Input: part model. Units: mm. Frame: model coordinates. A direction names the side the tool comes from. Round coordinates to 2 decimals unless told otherwise and drop trailing zeros. Loops run counter-clockwise (first coordinate to the right, second up) from the corner with the lowest first, then second, coordinate; pieces in that order, holes last. Notation, with made-up numbers: (55, 8) - (90, 8) arc R21 cw to (90, 32) - close; hole circle Ø8 at (11.25, 23.25). An arc over 180 degrees is marked (long way). One line per question, with ' | ' between items. Start each with the question number.
Item 1: Set-up query: faces 5 (the face through (-34.533, -0.493, 32.81)), 6 (the face through (29, -25, -39)). Return all of +Z, -Z, +X, -X, +Y, -Y with unobstructed straight access to the full face (end or side cutting, diameter ignored); none if empty.
Item 2: Section D-D, the plane y = -4. Return loops of the section in (x, z), plus the area to 3 significant figures.
Item 3: Draft query along Y for faces 1 (the face through (66.87, -61.5, -39.49)), 2 (the face through (-17, 0, -1)), 3 (the face through (57.751, -55.154, 39.507)), 4 (the face through (29, -25, -40)). Return one class per face: pulls with the +Y half, pulls with the -Y half, needs draft (parallel to the pull), parting line crosses it, or undercut.
Item 4: Section B-B, the plane z = 0. Return loops of the section in (x, y), plus the area to 3 significant figures.
Item 5: Section A-A, the plane x = -32.55. Return loops of the section in (y, z), plus the area to 3 significant figures.
Item 6: Section C-C, the plane z = -32.55. Return loops of the section in (x, y), plus the area to 3 significant figures.
Item 7: First-contact query: pin 1 (20 mm diameter, centred on x = 0, z = 0, fed in from +Y); pin 2 (5 mm diameter, centred on x = 32.55, z = -32.55, fed in from -Y); pin 3 (10.5 mm diameter, centred on x = 61.3, y = -57, fed in from -Z); pin 4 (1.6 mm diameter, centred on y = -0.5, z = -39, fed in from -X). Flat tips, straight axial feed; report the tip coordinate or a pass-through.
Item 8: Material intervals for line 1 along Z through (x, y) = (31.5, -24); line 2 along Y through (x, z) = (-23, 3); line 3 along X through (y, z) = (-57, -39.5), sorted ascending.
```python
from build123d import *

# Parameters (mm, degrees)
SKETCH2_W            = 76
SKETCH2_H            = 76
BASE_FLANGE1_DEPTH   = 1
SKETCH7_R            = 2
SKETCH7_R_2          = 16.65
CUT_EXTRUDE2_DEPTH   = 10
CIRPATTERN1_COUNT    = 4
EDGE_FLANGE1_DEPTH   = 50.083809579
SKETCH14_W           = 30.3
SKETCH14_H           = 61
TAB1_DEPTH           = 1
FILLET1_R            = 5
CUT_EXTRUDE4_DEPTH   = 10
CUT_EXTRUDE5_DEPTH   = 10
FILLET2_R            = 5
SKETCH19_R           = 4
CUT_EXTRUDE6_DEPTH   = 10
FILLET1_OF_MIRROR1_R = 5
FILLET2_OF_MIRROR1_R = 5


# Sheet-metal steps are written as plain solids
with BuildPart() as part:
    # Sketch2 → Base-Flange1 (new body)
    with BuildSketch(Plane(origin=(0, 0, 0), x_dir=(1, 0, 0), z_dir=(0, 1, 0))):
        Rectangle(SKETCH2_W, SKETCH2_H)
    extrude(amount=-BASE_FLANGE1_DEPTH)

    # Sketch7 → Cut-Extrude2 (cut)
    with BuildSketch(Plane(origin=(0, 0, 0), x_dir=(1, 0, 0), z_dir=(0, 1, 0))):
        with Locations(Location((32.55, 32.55, 0), (0, 0, 270))):
            Circle(SKETCH7_R)
        with Locations(Location((0, 0, 0), (0, 0, 270))):
            Circle(SKETCH7_R_2)
    cut_extrude2 = extrude(amount=-CUT_EXTRUDE2_DEPTH, mode=Mode.SUBTRACT)

    # CirPattern1: Cut-Extrude2 ×4 about axis
    cirpattern1_axis = Axis((0, 0, 0), (0, 1, 0))
    for i in range(1, CIRPATTERN1_COUNT):
        add(cut_extrude2.rotate(cirpattern1_axis, i * 360 / CIRPATTERN1_COUNT), mode=Mode.SUBTRACT)

    # Edge-Flange1 section (across the edge) → Edge-Flange1 (add)
    with BuildSketch(Plane(origin=(-12.083809579, -1, -39), x_dir=(0, 0, 1), z_dir=(1, 0, 0))):
        with BuildLine():
            Line((-1, 1), (-1, 62))
            Line((-1, 62), (0, 62))
            Line((0, 62), (0, 1))
            ThreePointArc((0, 1), (0.292893219, 0.292893219), (1, 0))
            Line((1, 0), (1, -1))
            ThreePointArc((1, -1), (-0.414213562, -0.414213562), (-1, 1))
        make_face()
    edge_flange1 = extrude(amount=EDGE_FLANGE1_DEPTH)

    # Sketch14 → Tab1 (add)
    with BuildSketch(Plane(origin=(0, 0, -40), x_dir=(-1, 0, 0), z_dir=(0, 0, -1))):
        with Locations((-53.15, -32.5)):
            Rectangle(SKETCH14_W, SKETCH14_H)
    tab1 = extrude(amount=-TAB1_DEPTH)

    # Fillet1
    fillet1_edges = [part.edges().sort_by_distance(p)[0] for p in [
        (68.3, -63, -39.5),
    ]]
    fillet(fillet1_edges, radius=FILLET1_R)

    # Sketch20 → Cut-Extrude4 (cut)
    with BuildSketch(Plane(origin=(0, 0, -40), x_dir=(-1, 0, 0), z_dir=(0, 0, -1))):
        Polygon((-38, -2), (-68.3, -54.482600826), (-68.3, -2), align=None)
    cut_extrude4 = extrude(amount=-CUT_EXTRUDE4_DEPTH, mode=Mode.SUBTRACT)

    # Sketch21 → Cut-Extrude5 (cut)
    with BuildSketch(Plane(origin=(0, 0, -40), x_dir=(-1, 0, 0), z_dir=(0, 0, -1))):
        Polygon((12.083809579, -2), (-55.544985759, -63), (12.083809579, -63), align=None)
    cut_extrude5 = extrude(amount=-CUT_EXTRUDE5_DEPTH, mode=Mode.SUBTRACT)

    # Fillet2
    fillet2_edges = [part.edges().sort_by_distance(p)[0] for p in [
        (55.544985759, -63, -39.5),
        (68.3, -54.482600826, -39.5),
    ]]
    fillet(fillet2_edges, radius=FILLET2_R)

    # Sketch19 → Cut-Extrude6 (cut)
    with BuildSketch(Plane(origin=(0, 0, -40), x_dir=(-1, 0, 0), z_dir=(0, 0, -1))):
        with Locations(Location((-61.3, -57, 0), (0, 0, 90))):
            Circle(SKETCH19_R)
    cut_extrude6 = extrude(amount=-CUT_EXTRUDE6_DEPTH, mode=Mode.SUBTRACT)

    # Mirror1: Edge-Flange1, Tab1, Cut-Extrude4, Cut-Extrude5, Cut-Extrude6 across plane
    add(edge_flange1.mirror(Plane.XY))
    add(tab1.mirror(Plane.XY))
    add(cut_extrude4.mirror(Plane.XY), mode=Mode.SUBTRACT)
    add(cut_extrude5.mirror(Plane.XY), mode=Mode.SUBTRACT)
    add(cut_extrude6.mirror(Plane.XY), mode=Mode.SUBTRACT)

    # Fillet1 of Mirror1
    fillet1_of_mirror1_edges = [part.edges().sort_by_distance(p)[0] for p in [
        (68.3, -63, 39.5),
    ]]
    fillet(fillet1_of_mirror1_edges, radius=FILLET1_OF_MIRROR1_R)

    # Fillet2 of Mirror1
    fillet2_of_mirror1_edges = [part.edges().sort_by_distance(p)[0] for p in [
        (55.544985759, -63, 39.5),
        (68.3, -54.482600826, 39.5),
    ]]
    fillet(fillet2_of_mirror1_edges, radius=FILLET2_OF_MIRROR1_R)


solid = part.part
```
Return value:
1) face 5: +Y, -Y | face 6: +X, -X, -Y
2) outline: (-9.87, -40) - (39.15, -40) - (39.15, -39) - (-9.87, -39) - close; (-9.87, 39) - (39.15, 39) - (39.15, 40) - (-9.87, 40) - close | area: 98.0 mm2
3) face 1: pulls with the -Y half | face 2: pulls with the +Y half | face 3: undercut | face 4: needs draft
4) outline: (-38, -1) - (-16.65, -1) - (-16.65, 0) - (-38, 0) - close; (16.65, -1) - (38, -1) - (38, 0) - (16.65, 0) - close | area: 42.7 mm2
5) outline: (-1, -38) - (0, -38) - (0, -34.55) - (-1, -34.55) - close; (-1, -30.55) - (0, -30.55) - (0, 30.55) - (-1, 30.55) - close; (-1, 34.55) - (0, 34.55) - (0, 38) - (-1, 38) - close | area: 68.0 mm2
6) outline: (-38, -1) - (-34.55, -1) - (-34.55, 0) - (-38, 0) - close; (-30.55, -1) - (30.55, -1) - (30.55, 0) - (-30.55, 0) - close; (34.55, -1) - (38, -1) - (38, 0) - (34.55, 0) - close | area: 68.0 mm2
7) pin 1: through | pin 2: y = -1 | pin 3: z = -40 | pin 4: x = -12.08
8) line 1: -40 to -39, 39 to 40 | line 2: -1 to 0 | line 3: 48.89 to 57.3, 65.3 to 68.3
